The model under review builds one solid part; all positions refer to its coordinate system, in mm. Coordinates: 2 decimals unless noted, no trailing zeros. Write each loop counter-clockwise with the first axis right and the second up, starting at its lowest first coordinate (ties: lowest second). Pieces come first, ordered by that corner, then holes. Notation, with made-up numbers: (80, -0.75) - (108, -0.75) arc R15 cw to (108, 26.25) - close; hole circle Ø8 at (84.25, -23.75). An arc over 180 degrees is marked (long way). Put each result on its own line as item: value. Start each with the question number.
Item 1: To check wall thickness, follow L1, parallel to X at y = -33, z = 0.35; L2, parallel to Y at x = -65, z = 0.9; L3, parallel to X at y = -3.5, z = 1.5. State the ranges of each line that lie inside material, in increasing order. Write a range as [from, to].
Item 2: Consider section B-B on x = 42. Give the boundary of the cut face in (y, z) (3 decimals).
Item 3: Consider section A-A on y = 0. Give the boundary of the cut face in (x, z) (3 decimals), then the cut area to 3 significant figures.
Item 4: Consider section C-C on x = 0. Give the boundary of the cut face in (y, z) (3 decimals), then the cut area to 3 significant figures.
Item 5: Consider section D-D on y = -18. Give the boundary of the cut face in (x, z) (3 decimals), then the cut area to 3 significant figures.
Item 6: For pin 1 (5 mm diameter, centred on x = 0, y = 38.1, fed in from -Z); pin 2 (2.5 mm diameter, centred on x = 66.675, y = 34.925, fed in from -Z), all flat-tipped, find the tip position at first contact; note any pin that passes through.
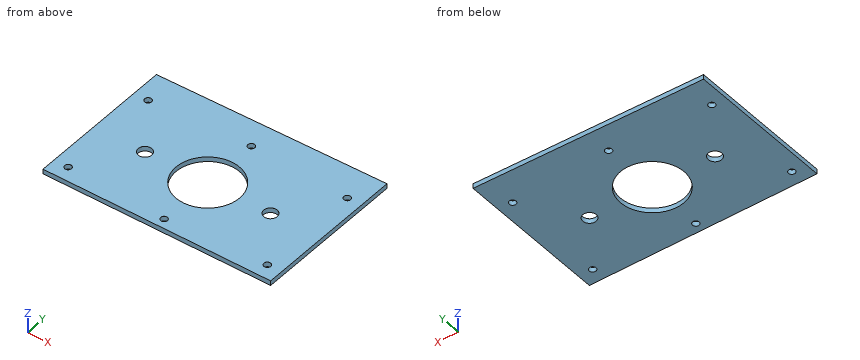
```python
from build123d import *

# Parameters (mm, degrees)
BOSS_EXTRUDE1_DEPTH            = 3.175
M4_CLEARANCE_HOLE1_D           = 4.5
M4_CLEARANCE_HOLE1_CSINK_D     = 4.55
M4_CLEARANCE_HOLE1_CSINK_ANGLE = 90
M8_CLEARANCE_HOLE1_AT_2_COUNT  = 2
M8_CLEARANCE_HOLE1_AT_2_PITCH  = 84
SKETCH9_R                      = 21.275
CENTER_HOLE_DEPTH              = 96.302901976


with BuildPart() as part:
    # Sketch1 → Boss-Extrude1 (new body)
    with BuildSketch(Plane.XY):
        Polygon((-76.2, 54.61), (-76.2, 44.45), (-76.2, -44.45), (76.2, -44.45), (76.2, 44.45), (76.2, 57.15), align=None)
    extrude(amount=BOSS_EXTRUDE1_DEPTH)

    # M4 Clearance Hole1 (through all)
    with Locations(Plane.XY.offset(3.175)):
        with Locations((0, 38.1), (-66.675, 34.925), (-66.675, -34.925), (0, -38.1), (66.675, -34.925), (66.675, 34.925)):
            CounterSinkHole(M4_CLEARANCE_HOLE1_D / 2, M4_CLEARANCE_HOLE1_CSINK_D / 2, counter_sink_angle=M4_CLEARANCE_HOLE1_CSINK_ANGLE)

    # Sketch11 → M8 Clearance Hole1 (revolve, cut)
    with BuildSketch(Plane(origin=(-42, 0, 3.175), x_dir=(0, -1, 0), z_dir=(1, 0, 0))):
        Polygon((0, 0), (0, 3.175), (4.5, 3.175), (4.5, 0.025), (4.525, 0), align=None)
    m8_clearance_hole1 = revolve(axis=Axis((-42, 0, 9.525), (0, 0, -1)), mode=Mode.SUBTRACT)

    # M8 Clearance Hole1 at 2: M8 Clearance Hole1 ×2
    with Locations(*[(i * M8_CLEARANCE_HOLE1_AT_2_PITCH, 0, 0) for i in range(1, M8_CLEARANCE_HOLE1_AT_2_COUNT)]):
        add(m8_clearance_hole1, mode=Mode.SUBTRACT)

    # Sketch9 → Center Hole (cut, through all)
    with BuildSketch(Plane.XY.offset(3.175)):
        Circle(SKETCH9_R)
    extrude(amount=-CENTER_HOLE_DEPTH, mode=Mode.SUBTRACT)


solid = part.part
```
Report:
1. L1: [-76.2, -67.84], [-65.51, 65.51], [67.84, 76.2]
1. L2: [-44.45, -36.43], [-33.42, 33.42], [36.43, 54.8]
1. L3: [-76.2, -44.83], [-39.17, -20.99], [20.99, 39.17], [44.83, 76.2]
2. outline: (-44.45, 0) - (-4.5, 0) - (-4.5, 3.15) - (-4.525, 3.175) - (-44.45, 3.175) - close; (4.5, 0) - (56.58, 0) - (56.58, 3.175) - (4.525, 3.175) - (4.5, 3.15) - close
3. outline: (-76.2, 0) - (-46.5, 0) - (-46.5, 3.15) - (-46.525, 3.175) - (-76.2, 3.175) - close; (-37.5, 0) - (-21.275, 0) - (-21.275, 3.175) - (-37.475, 3.175) - (-37.5, 3.15) - close; (21.275, 0) - (37.5, 0) - (37.5, 3.15) - (37.475, 3.175) - (21.275, 3.175) - close; (46.5, 0) - (76.2, 0) - (76.2, 3.175) - (46.525, 3.175) - (46.5, 3.15) - close
3. area: 292 mm²
4. outline: (-44.45, 0) - (-40.35, 0) - (-40.35, 3.15) - (-40.375, 3.175) - (-44.45, 3.175) - close; (-35.85, 0) - (-21.275, 0) - (-21.275, 3.175) - (-35.825, 3.175) - (-35.85, 3.15) - close; (21.275, 0) - (35.85, 0) - (35.85, 3.15) - (35.825, 3.175) - (21.275, 3.175) - close; (40.35, 0) - (55.88, 0) - (55.88, 3.175) - (40.375, 3.175) - (40.35, 3.15) - close
4. area: 155 mm²
5. outline: (-76.2, 0) - (-11.341, 0) - (-11.341, 3.175) - (-76.2, 3.175) - close; (11.341, 0) - (76.2, 0) - (76.2, 3.175) - (11.341, 3.175) - close
5. area: 412 mm²
6. pin 1: z = 0
6. pin 2: through
